The figure shows three views and two pictorial views of one solid part (mm, origin at its lowest corner). Answer the questions. A direction names the side the tool comes from. Coordinates: 2 decimals unless noted, no trailing zeros. Write each loop counter-clockwise with the first axis right and the second up, starting at its lowest first coordinate (ties: lowest second). Pieces come first, ordered by that corner, then holes. Notation, with made-up numbers: (-14, 62) - (8, 62) arc R14 ccw to (8, 76) - close; hole circle Ø3 at (-6, 28.5). An arc over 180 degrees is marked (long way). Use a Markdown table: item, result. Add a question column.
(1) For a pull along Z with two mould halves and no side action, classify the marked faces 4, 5, 6 and 7 as released by +Z, released by -Z, zero draft, split by the parting line, or undercut.
(2) The part is cut by section C-C, the plane y = 0.95. Give the vertices of the cut face in (x, z).
(3) The part is cut by section B-B, the plane z = 3.5. Give the vertices of the cut face in (x, y), then the cut area to 3 significant figures.
(4) The part is cut by section D-D, the plane x = 12.25. Give the vertices of the cut face in (y, z).
(5) The part is cut by section A-A, the plane x = 3. Give the vertices of the cut face in (y, z), then the cut area to 3 significant figures.
(6) Find the intervals of material crossed by line 1 (X direction, y = 0.55, z = 3.5); line 2 (Y direction, x = 15.5, z = 10.25); line 3 (Z direction, x = 19.75, y = 0.3), in increasing order. Write a range as from..to.
(7) Given pin 1 Ø3.5 at (x, z) = (18, 3.5) entering from -Y; pin 2 Ø3 at (x, y) = (9.5, 4) entering from +Z; pin 3 Ø1 at (y, z) = (3.5, 4) entering from -X; pin 4 Ø1.6 at (x, y) = (13, 0.5) entering from -Z, each flat-ended and moving along its own axis, determine where each tip first touches the part or whether it passes through.
(8) A tool of negligible diameter and unlimited length cuts with its end or side. For the marked faces 1, 2 and 3, from which of +Z, -Z, +X, -X, +Y, -Y can it reach the whole face along a straight path? Write none if from no direction.
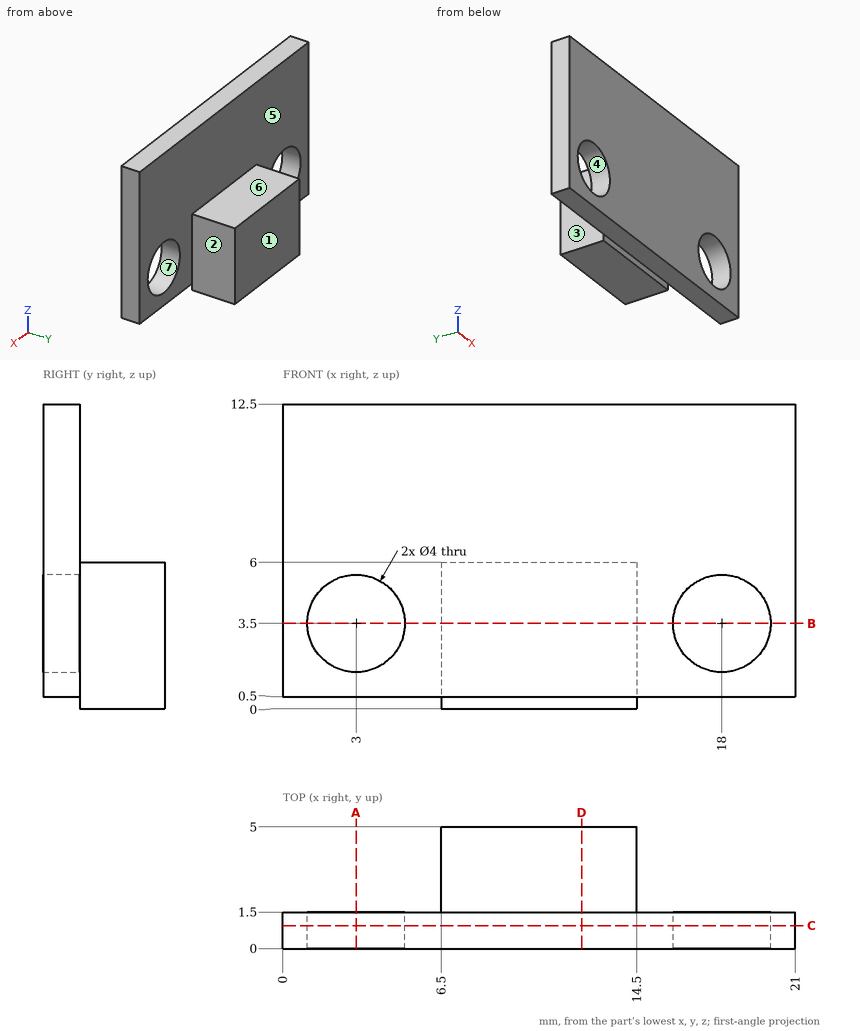
Model answer:
| question | item | result |
|---|---|---|
| 1 | face 4 | undercut |
| 1 | face 5 | zero draft |
| 1 | face 6 | released by +Z |
| 1 | face 7 | undercut |
| 2 | outline | (0, 0.5) - (21, 0.5) - (21, 12.5) - (0, 12.5) - close; hole circle Ø4 at (3, 3.5); hole circle Ø4 at (18, 3.5) |
| 3 | outline | (0, 0) - (1, 0) - (1, 1.5) - (0, 1.5) - close; (5, 0) - (16, 0) - (16, 1.5) - (14.5, 1.5) - (14.5, 5) - (6.5, 5) - (6.5, 1.5) - (5, 1.5) - close; (20, 0) - (21, 0) - (21, 1.5) - (20, 1.5) - close |
| 3 | area | 47.5 mm^2 |
| 4 | outline | (0, 0.5) - (1.5, 0.5) - (1.5, 0) - (5, 0) - (5, 6) - (1.5, 6) - (1.5, 12.5) - (0, 12.5) - close |
| 5 | outline | (0, 0.5) - (1.5, 0.5) - (1.5, 1.5) - (0, 1.5) - close; (0, 5.5) - (1.5, 5.5) - (1.5, 12.5) - (0, 12.5) - close |
| 5 | area | 12.0 mm^2 |
| 6 | line 1 | 0..1, 5..16, 20..21 |
| 6 | line 2 | 0..1.5 |
| 6 | line 3 | 0.5..2.53, 4.47..12.5 |
| 7 | pin 1 | through |
| 7 | pin 2 | z = 6 |
| 7 | pin 3 | x = 6.5 |
| 7 | pin 4 | z = 0.5 |
| 8 | face 1 | +Z, -Z, +X, -X, +Y |
| 8 | face 2 | +Z, -Z, +X, +Y |
| 8 | face 3 | +Z, -Z, -X, +Y |
